Check sheet for the modelled part. Datum: model origin and axes. Units: mm. A direction names the side the tool comes from. Give positions to 0.01 mm unless a question says otherwise; leave off trailing zeros. Write each loop counter-clockwise with the first axis right and the second up, starting at its lowest first coordinate (ties: lowest second). Pieces come first, ordered by that corner, then holes. Notation, with made-up numbers: (18.25, 67) -> (58.25, 67) arc R19 ccw to (58.25, 92) -> close; hole circle Ø2 at (86.5, 35.25). An arc over 180 degrees is marked (long way). Return JSON: item names as keys, results as strings.
from build123d import *

# Parameters (mm, degrees)
F0_W     = 7.9375
F0_H     = 7.9375
F1_DEPTH = 9.525
F2_R     = 2.4257
F3_DEPTH = 1.778
F4_W     = 5.7531
F4_H     = 5.7531
F5_DEPTH = 8.4328


with BuildPart() as f1:
    # F0 (on Top) → F1 (new body)
    with BuildSketch(Plane.XY):
        with Locations((-18.788291, 11.73261)):
            Rectangle(F0_W, F0_H)
    extrude(amount=F1_DEPTH)

    # F2 (on face) → F3 (join)
    with BuildSketch(Plane.XY.offset(9.525)):
        with Locations((-18.794646, 11.738965)):
            Circle(F2_R)
    extrude(amount=F3_DEPTH)

    # F4 (on face) → F5 (cut)
    with BuildSketch(Plane(origin=(0, 0, 0), x_dir=(1, 0, 0), z_dir=(0, 0, -1))):
        with Locations((-18.788291, -11.73261)):
            Rectangle(F4_W, F4_H)
    extrude(amount=-F5_DEPTH, mode=Mode.SUBTRACT)


solid = f1.part
(1) Cross-section at A-A on z = 5. Enter the section's corners in (x, y), then the cut area to 3 significant figures.
Reply:
{"outline": "(-22.76, 7.76) -> (-14.82, 7.76) -> (-14.82, 15.7) -> (-22.76, 15.7) -> close; hole (-21.66, 8.86) -> (-15.91, 8.86) -> (-15.91, 14.61) -> (-21.66, 14.61) -> close", "area": "29.9 mm^2"}
(2) Cross-section at C-C on x = -15.75. Enter the section's corners in (y, z) (3 decimals).
Reply:
{"outline": "(7.764, 0) -> (15.701, 0) -> (15.701, 9.525) -> (7.764, 9.525) -> close"}
(3) Release check for a two-part mould opening along X. For faces 1 (the flat face through (-15, 12, 0)), 2 (the flat face through (-19, 8.856, 4)), 3 (the flat face through (-22.757, 12, 5)), 4 (the cylindrical face through (-16.48, 12.47, 10.4)) record: pulls with the +X half, pulls with the -X half, needs draft (parallel to the pull), parting line crosses it, or undercut.
Reply:
{"face 1": "needs draft", "face 2": "undercut", "face 3": "pulls with the -X half", "face 4": "parting line crosses it"}
(4) Cross-section at B-B on y = 9.5. Enter the section's corners in (x, z) (3 decimals), then the cut area to 3 significant figures.
Reply:
{"outline": "(-22.757, 0) -> (-21.665, 0) -> (-21.665, 8.433) -> (-15.912, 8.433) -> (-15.912, 0) -> (-14.82, 0) -> (-14.82, 9.525) -> (-17.861, 9.525) -> (-17.861, 11.303) -> (-19.728, 11.303) -> (-19.728, 9.525) -> (-22.757, 9.525) -> close", "area": "30.4 mm^2"}
(5) Thickness scan on L1, parallel to X at y = 13, z = 6.5; L2, parallel to Y at x = -18, z = 4; L3, parallel to Z at x = -21, y = 13.25 (3 decimals). Record the ranges inside material, lowest first.
Reply:
{"L1": "-22.76 to -21.66, -15.91 to -14.82", "L2": "7.76 to 8.86, 14.61 to 15.7", "L3": "8.433 to 9.525"}
(6) Cross-section at D-D on y = 15.25. Enter the section's corners in (x, z) (3 decimals), then the cut area to 3 significant figures.
Reply:
{"outline": "(-22.757, 0) -> (-14.82, 0) -> (-14.82, 9.525) -> (-22.757, 9.525) -> close", "area": "75.6 mm^2"}
(7) Set-up check for faces 5 (the flat face through (-19, 14.609, 4)), 6 (the flat face through (-21, 14, 9.525)), 7 (the flat face through (-19, 12, 11.303)): record each of +Z, -Z, +X, -X, +Y, -Y from which the full face is reachable in a straight line by a thin tool's end or side.
Reply:
{"face 5": "-Z", "face 6": "+Z", "face 7": "+Z, +X, -X, +Y, -Y"}
